from build123d import *

# Parameters (mm, degrees)
EXTRUDE_START                      = 0.2
EXTRUDE_1_DEPTH                    = 5.1
SKETCH_7_W                         = 0.3
SKETCH_7_H                         = 0.2
EXTRUDE_4_DEPTH                    = 11.5
SKETCH_8_W                         = 1
SKETCH_8_H                         = 2
CUT_EXTRUDE_5_DEPTH                = 8.57
CUT_EXTRUDE_1_DEPTH                = 9.2
EXTRUDE_2_DEPTH                    = 3.8
SKETCH_4_W                         = 5.63
SKETCH_4_H                         = 1
CUT_EXTRUDE_2_DEPTH                = 3.8
CUT_EXTRUDE_3_REACH                = 17.485
CHAMFER_1_SIZE                     = 0.5
CUT_EXTRUDE_6_REACH                = 16.449
SKETCH_9_W                         = 0.7
SKETCH_9_H                         = 1
SWEEP_START                        = 2.22
SWEEP_1_DEPTH                      = 0.64
CHAMFER_2_SIZE                     = 0.2
PATTERN_LINEAR_2_COUNT             = 3
PATTERN_LINEAR_2_PITCH             = 2.54
PATTERN_LINEAR_1_COUNT             = 3
PATTERN_LINEAR_1_PITCH             = 2.54
CHAMFER_2_OF_PATTERN_LINEAR_1_SIZE = 0.2


# Read off the part's stored shape, not the designer's step: По траектории1
with BuildPart() as part:
    # Эскиз1 → Бобышка-Вытянуть1 (new body)
    with BuildSketch(Plane.XY.offset(EXTRUDE_START)):
        Polygon((-4.285, 0.55), (4.285, 0.55), (4.285, -1.45), (5.085, -1.45), (5.085, -12.95), (-5.085, -12.95), (-5.085, -1.45), (-4.285, -1.45), align=None)
    extrude(amount=EXTRUDE_1_DEPTH)

    # Эскиз7 → Бобышка-Вытянуть4 (add)
    with BuildSketch(Plane.XZ.offset(12.95)):
        with Locations((3.535, 0.1)):
            Rectangle(SKETCH_7_W, SKETCH_7_H)
        with Locations((-3.535, 0.1)):
            Rectangle(SKETCH_7_W, SKETCH_7_H)
    extrude(amount=-EXTRUDE_4_DEPTH)

    # Эскиз8 → Вырез-Вытянуть5 (cut)
    with BuildSketch(Plane(origin=(4.285, 0, 0), x_dir=(0, 0, -1), z_dir=(1, 0, 0))):
        with Locations((-0.7, -0.45)):
            Rectangle(SKETCH_8_W, SKETCH_8_H)
        Polygon((-4.2, -1.45), (-5.3, -1.45), (-5.3, 0.55), (-3.9, 0.55), (-3.9, -0.45), (-4.2, -0.45), align=None)
    extrude(amount=-CUT_EXTRUDE_5_DEPTH, mode=Mode.SUBTRACT)

    # Эскиз2 → Вырез-Вытянуть1 (cut)
    with BuildSketch(Plane.XZ.offset(12.95)):
        Polygon((-4.085, 4.3), (-4.085, 1.2), (0.67, 1.2), (0.67, 0.2), (1.87, 0.2), (1.87, 1.2), (4.085, 1.2), (4.085, 4.3), (1.5, 4.3), (1.5, 5.3), (-1.5, 5.3), (-1.5, 4.3), align=None)
    extrude(amount=-CUT_EXTRUDE_1_DEPTH, mode=Mode.SUBTRACT)

    # Эскиз3 → Бобышка-Вытянуть2 (add)
    with BuildSketch(Plane.XZ.offset(12.95)):
        Polygon((-3.815, 5.3), (-3.815, 6.8), (3.815, 6.8), (3.815, 5.3), (2.815, 5.3), (2.815, 5.8), (-2.815, 5.8), (-2.815, 5.3), align=None)
    extrude(amount=-EXTRUDE_2_DEPTH)

    # Эскиз4 → Вырез-Вытянуть2 (cut)
    with BuildSketch(Plane.XZ.offset(12.95)):
        with Locations((0, 4.8)):
            Rectangle(SKETCH_4_W, SKETCH_4_H)
    extrude(amount=-CUT_EXTRUDE_2_DEPTH, mode=Mode.SUBTRACT)

    # Эскиз5 → Вырез-Вытянуть3 (cut, up to next)
    with BuildSketch(Plane.XY.offset(6.8), mode=Mode.PRIVATE) as cut_extrude_3_sk1:
        with BuildLine():
            Line((2.815, -9.15), (2.815, -10.95))
            ThreePointArc((2.815, -10.95), (2.668553391, -11.303553391), (2.315, -11.45))
            Line((2.315, -11.45), (-2.315, -11.45))
            ThreePointArc((-2.315, -11.45), (-2.668553391, -11.303553391), (-2.815, -10.95))
            Line((-2.815, -10.95), (-2.815, -9.15))
            Line((-2.815, -9.15), (2.815, -9.15))
        make_face()
    cut_extrude_3_tool1 = extrude(cut_extrude_3_sk1.sketch, amount=-CUT_EXTRUDE_3_REACH, mode=Mode.PRIVATE) & part.part
    add(cut_extrude_3_tool1.solids().sort_by_distance((0, -10.291324, 6.8))[0], mode=Mode.SUBTRACT)

    # Фаска1
    chamfer_1_edges = [part.edges().sort_by_distance(p)[0] for p in [
        (-2.815, -12.95, 5.05),
        (0, -12.95, 5.8),
        (2.815, -12.95, 5.05),
        (2.1575, -9.15, 4.3),
        (-3.45, -12.95, 4.3),
        (-2.1575, -9.15, 4.3),
        (-4.085, -12.95, 2.75),
        (-1.7075, -12.95, 1.2),
        (2.9775, -12.95, 1.2),
        (4.085, -12.95, 2.75),
        (3.45, -12.95, 4.3),
    ]]
    chamfer(chamfer_1_edges, length=CHAMFER_1_SIZE)

    # Эскиз9 → Вырез-Вытянуть6 (cut, up to next)
    with BuildSketch(Plane.XY.offset(3.9), mode=Mode.PRIVATE) as cut_extrude_6_sk1:
        with Locations((2.545, 0.05)):
            Rectangle(SKETCH_9_W, SKETCH_9_H)
    cut_extrude_6_tool1 = extrude(cut_extrude_6_sk1.sketch, amount=-CUT_EXTRUDE_6_REACH, mode=Mode.PRIVATE) & part.part
    cut_extrude_6 = cut_extrude_6_tool1.solids().sort_by_distance((2.545, 0.05, 3.9))[0]
    add(cut_extrude_6, mode=Mode.SUBTRACT)

    # По траектории1 outline → По траектории1 (add)
    with BuildSketch(Plane.YZ.offset(SWEEP_START)):
        with BuildLine():
            Line((-3.75, 2.43), (-3.75, 3.07))
            add(Edge.make_bspline(
                [(-3.75, 3.07), (-4.166666667, 3.07), (-4.583333333, 3.07), (-6.516666667, 3.07), (-8.033333333, 3.07), (-9.55, 3.07)],
                knots=[0.623544277, 0.623544277, 0.623544277, 0.623544277, 0.704676976, 0.704676976, 1, 1, 1, 1], degree=3))
            Line((-9.55, 3.07), (-9.55, 2.43))
            Line((-9.55, 2.43), (-3.75, 2.43))
        make_face()
        with BuildLine():
            Line((0.32, -3.3), (0.32, 2.3))
            add(Edge.make_bspline(
                [(0.32, 2.3), (0.32, 2.499654349), (0.23877091, 2.700173533), (0.022322877, 2.916621566), (-0.064240468, 2.973940923), (-0.250203983, 3.050392149), (-0.370157621, 3.069944018), (-0.45, 3.07)],
                knots=[0.363474491, 0.363474491, 0.363474491, 0.363474491, 0.386414221, 0.386414221, 0.397884087, 0.397884087, 0.409353952, 0.409353952, 0.409353952, 0.409353952], degree=3))
            Line((-0.45, 3.07), (-0.45, 2.43))
            ThreePointArc((-0.45, 2.43), (-0.358076118, 2.391923882), (-0.32, 2.3))
            Line((-0.32, 2.3), (-0.32, -3.3))
            Line((-0.32, -3.3), (0.32, -3.3))
        make_face()
    sweep_1 = extrude(amount=SWEEP_1_DEPTH)

    # Фаска2
    chamfer_2_edges = [part.edges().sort_by_distance(p)[0] for p in [
        (2.54, -9.55, 3.07),
        (2.86, -9.55, 2.75),
        (2.54, -9.55, 2.43),
        (2.22, -9.55, 2.75),
        (2.54, -0.32, -3.3),
        (2.86, 0, -3.3),
        (2.54, 0.32, -3.3),
        (2.22, 0, -3.3),
    ]]
    chamfer(chamfer_2_edges, length=CHAMFER_2_SIZE)

    # Линейный массив2: Вырез-Вытянуть6 ×3
    with Locations(*[(-i * PATTERN_LINEAR_2_PITCH, 0, 0) for i in range(1, PATTERN_LINEAR_2_COUNT)]):
        add(cut_extrude_6, mode=Mode.SUBTRACT)

    # Линейный массив1: По траектории1 ×3
    with Locations(*[(-i * PATTERN_LINEAR_1_PITCH, 0, 0) for i in range(1, PATTERN_LINEAR_1_COUNT)]):
        add(sweep_1)

    # Фаска2 of Линейный массив1
    chamfer_2_of_pattern_linear_1_edges = [part.edges().sort_by_distance(p)[0] for p in [
        (0, -9.55, 3.07),
        (0.32, -9.55, 2.75),
        (0, -9.55, 2.43),
        (-0.32, -9.55, 2.75),
        (0, -0.32, -3.3),
        (0.32, 0, -3.3),
        (0, 0.32, -3.3),
        (-0.32, 0, -3.3),
        (-2.54, -9.55, 3.07),
        (-2.22, -9.55, 2.75),
        (-2.54, -9.55, 2.43),
        (-2.86, -9.55, 2.75),
        (-2.54, -0.32, -3.3),
        (-2.22, 0, -3.3),
        (-2.54, 0.32, -3.3),
        (-2.86, 0, -3.3),
    ]]
    chamfer(chamfer_2_of_pattern_linear_1_edges, length=CHAMFER_2_OF_PATTERN_LINEAR_1_SIZE)


solid = part.part
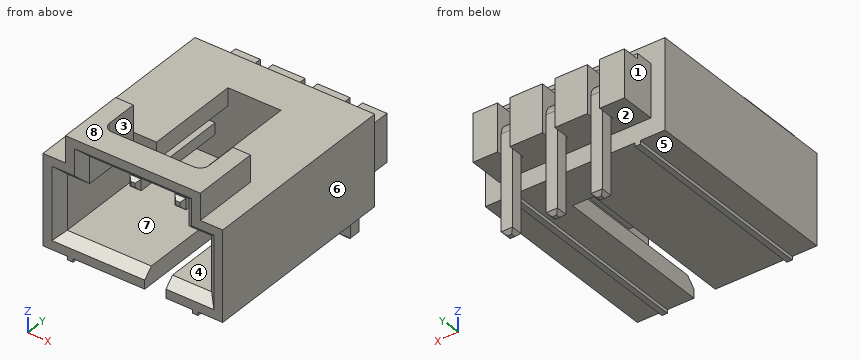
For this review, take the finished solid that the model builds, in its own axes (mm). Face numbers are marked on the shaded views. A direction names the side the tool comes from. Coordinates: 2 decimals unless noted, no trailing zeros. Order: outer loops, then holes, each group sorted by start corner. A loop starts at its lowest first (then second) coordinate and runs counter-clockwise, first axis right, second up. Notation, with made-up numbers: (11, 51.25) -> (16, 51.25) arc R20 cw to (16, 84.25) -> close; hole circle Ø1 at (-8.5, 80.25). An arc over 180 degrees is marked (long way). Return JSON: item names as keys, results as strings.
1. Machinability: for the marked faces 1, 2, 3 and 4, which of the approach directions +Z, -Z, +X, -X, +Y, -Y give a long, thin tool a straight path to every point of the face, cutting with its end or side? Answer none if there is none.
Answer block:
{"face 1": "+Z, -Z, -X, +Y", "face 2": "-Z", "face 3": "none", "face 4": "-Y"}
2. We need section B-B on z = -1.75. Write out the cut boundary in (x, y), and give its area (3 significant figures).
Answer block:
{"outline": "(-2.86, -0.32) -> (-2.22, -0.32) -> (-2.22, 0.32) -> (-2.86, 0.32) -> close; (-0.32, -0.32) -> (0.32, -0.32) -> (0.32, 0.32) -> (-0.32, 0.32) -> close; (2.22, -0.32) -> (2.86, -0.32) -> (2.86, 0.32) -> (2.22, 0.32) -> close", "area": "1.23 mm²"}
3. The part is to be moulded in two halves that separate along Z. For the marked faces 5, 6, 7 and 8, say which applies: +Z half, -Z half, draft (parallel to the pull), parting line (faces both ways), or undercut.
Answer block:
{"face 5": "-Z half", "face 6": "draft", "face 7": "undercut", "face 8": "+Z half"}
4. We need section C-C on y = -10.75. Write out the cut boundary in (x, z) (3 decimals), and give its area (3 significant figures).
Answer block:
{"outline": "(-5.085, 0.2) -> (-3.685, 0.2) -> (-3.685, 0) -> (-3.385, 0) -> (-3.385, 0.2) -> (0.67, 0.2) -> (0.67, 1.2) -> (-4.085, 1.2) -> (-4.085, 4.3) -> (-2.815, 4.3) -> (-2.815, 6.8) -> (-3.815, 6.8) -> (-3.815, 5.3) -> (-5.085, 5.3) -> close; (1.87, 0.2) -> (3.385, 0.2) -> (3.385, 0) -> (3.685, 0) -> (3.685, 0.2) -> (5.085, 0.2) -> (5.085, 5.3) -> (3.815, 5.3) -> (3.815, 6.8) -> (2.815, 6.8) -> (2.815, 4.3) -> (4.085, 4.3) -> (4.085, 1.2) -> (1.87, 1.2) -> close", "area": "22.8 mm²"}
5. For line 1 (X direction, y = -0.25, z = 1); line 2 (X direction, y = -4.75, z = 1.5) (3 decimals); line 3 (X direction, y = -4.25, z = 5) (3 decimals), list the stretches that pass through material, from the lowest coordinate up. Write a range as from..to.
Answer block:
{"line 1": "-2.86..-2.22, -0.32..0.32, 2.22..2.86", "line 2": "-5.085..-4.085, 4.085..5.085", "line 3": "-5.085..-1.5, 1.5..5.085"}
6. We need section A-A on x = -1. Write out the cut boundary in (y, z).
Answer block:
{"outline": "(-12.95, 0.2) -> (-1.45, 0.2) -> (-1.45, 1.2) -> (0.55, 1.2) -> (0.55, 3.9) -> (-0.45, 3.9) -> (-0.45, 4.2) -> (-1.45, 4.2) -> (-1.45, 5.3) -> (-3.75, 5.3) -> (-3.75, 1.2) -> (-12.45, 1.2) -> (-12.95, 0.7) -> close; (-12.95, 6.3) -> (-12.45, 5.8) -> (-11.45, 5.8) -> (-11.45, 6.8) -> (-12.95, 6.8) -> close"}
7. For pin 1 Ø2 at (x, y) = (2.5, -9.5) entering from -Z; pin 2 Ø1.1 at (x, z) = (-0.5, 6.5) entering from +Y; pin 3 Ø0.8 at (y, z) = (0, -1) entering from -X, all flat-tipped, find the tip position at first contact; note any pin that passes through.
Answer block:
{"pin 1": "z = 0", "pin 2": "y = -11.45", "pin 3": "x = -2.86"}
8. We need section D-D on y = -3.25. Write out the cut boundary in (x, z) (3 decimals).
Answer block:
{"outline": "(-5.085, 0.2) -> (-3.685, 0.2) -> (-3.685, 0) -> (-3.385, 0) -> (-3.385, 0.2) -> (3.385, 0.2) -> (3.385, 0) -> (3.685, 0) -> (3.685, 0.2) -> (5.085, 0.2) -> (5.085, 5.3) -> (-5.085, 5.3) -> close"}
